Model file for the job. Use its own axes, mm. A direction names the side the tool comes from. Round coordinates to 2 decimals unless told otherwise and drop trailing zeros. Loops run counter-clockwise (first coordinate to the right, second up) from the corner with the lowest first, then second, coordinate; pieces in that order, holes last. Notation, with made-up numbers: (-2.75, 22) - (12.25, 22) arc R14 cw to (12.25, 42) - close; hole circle Ø8 at (-11.5, 54.25). An arc over 180 degrees is marked (long way). Answer as a JSON object with one key per item and string values.
from build123d import *

# Parameters (mm, degrees)
SKETCH1_W                   = 76.1
SKETCH1_H                   = 151.5
BOSS_EXTRUDE2_DEPTH         = 8
SKETCH1_4_W                 = 76.1
SKETCH1_4_H                 = 3
BOSS_EXTRUDE3_DEPTH         = 18.5
CUT_EXTRUDE_THIN1_START     = -8
CUT_EXTRUDE_THIN1_OUTLINE_W = 50
CUT_EXTRUDE_THIN1_OUTLINE_H = 4.46993239
CUT_EXTRUDE_THIN1_DEPTH     = 18.5
SKETCH4_W                   = 76.1
SKETCH4_H                   = 3
CUT_EXTRUDE1_DEPTH          = 16.5
SKETCH6_W                   = 154.5
SKETCH6_H                   = 2
BOSS_EXTRUDE4_DEPTH         = 3
SKETCH7_W                   = 154.5
SKETCH7_H                   = 2
BOSS_EXTRUDE5_DEPTH         = 3
CUT_EXTRUDE2_DEPTH          = 3
CUT_EXTRUDE2_DEPTH_BACK     = 76.1
SKETCH8_R                   = 1.75


# Read off the part's stored shape, not the designer's step: Cut-Extrude-Thin1
with BuildPart() as part:
    # Sketch1 → Boss-Extrude2 (new body)
    with BuildSketch(Plane(origin=(0, 0, 0), x_dir=(1, 0, 0), z_dir=(0, 1, 0))):
        with Locations((38.05, -75.75)):
            Rectangle(SKETCH1_W, SKETCH1_H)
    extrude(amount=BOSS_EXTRUDE2_DEPTH)

    # Sketch1<4> → Boss-Extrude3 (add)
    with BuildSketch(Plane(origin=(0, 0, 0), x_dir=(1, 0, 0), z_dir=(0, 1, 0))):
        Polygon((0, -151.5), (-3, -151.5), (-3, -155.96993239), (79.1, -155.96993239), (79.1, -151.5), (76.1, -151.5), align=None)
        Polygon((0, 3), (-3, 3), (-3, -151.5), (0, -151.5), (0, 0), align=None)
        Polygon((79.1, 3), (79.1, -151.5), (76.1, -151.5), (76.1, 0), (76.1, 3), align=None)
        with Locations((38.05, 1.5)):
            Rectangle(SKETCH1_4_W, SKETCH1_4_H)
    extrude(amount=BOSS_EXTRUDE3_DEPTH)

    # Cut-Extrude-Thin1 outline → Cut-Extrude-Thin1 (cut)
    with BuildSketch(Plane(origin=(0, 8, 0), x_dir=(1, 0, 0), z_dir=(0, 1, 0)).offset(CUT_EXTRUDE_THIN1_START)):
        with Locations((38.05, -153.734966195)):
            Rectangle(CUT_EXTRUDE_THIN1_OUTLINE_W, CUT_EXTRUDE_THIN1_OUTLINE_H)
    extrude(amount=CUT_EXTRUDE_THIN1_DEPTH, mode=Mode.SUBTRACT)

    # Sketch4 → Cut-Extrude1 (cut)
    with BuildSketch(Plane(origin=(0, 18.5, 0), x_dir=(1, 0, 0), z_dir=(0, 1, 0))):
        with Locations((38.05, 1.5)):
            Rectangle(SKETCH4_W, SKETCH4_H)
    extrude(amount=-CUT_EXTRUDE1_DEPTH, mode=Mode.SUBTRACT)

    # Sketch6 → Boss-Extrude4 (add)
    with BuildSketch(Plane(origin=(0, 0, 0), x_dir=(0, 0, -1), z_dir=(1, 0, 0))):
        with Locations((-74.25, 17.5)):
            Rectangle(SKETCH6_W, SKETCH6_H)
    extrude(amount=BOSS_EXTRUDE4_DEPTH)

    # Sketch7 → Boss-Extrude5 (add)
    with BuildSketch(Plane.ZY.offset(-76.1)):
        with Locations((74.25, 17.5)):
            Rectangle(SKETCH7_W, SKETCH7_H)
    extrude(amount=BOSS_EXTRUDE5_DEPTH)

    # Sketch8 → Cut-Extrude2 (cut, two sides: drawn at the far end of the back side and taken through both)
    with BuildSketch(Plane(origin=(0, 8, 0), x_dir=(1, 0, 0), z_dir=(0, 1, 0)).offset(-CUT_EXTRUDE2_DEPTH_BACK)):
        with Locations(Location((38.05, -75.75, 0), (0, 0, 270))):
            Circle(SKETCH8_R)
    extrude(amount=CUT_EXTRUDE2_DEPTH + CUT_EXTRUDE2_DEPTH_BACK, mode=Mode.SUBTRACT)


solid = part.part
1) Slice it at D-D on x = 24. List the corners of the cut face in (y, z), then the cut area to 3 significant figures.
Values follow:
{"outline": "(0, -3) - (2, -3) - (2, 0) - (8, 0) - (8, 151.5) - (0, 151.5) - close", "area": "1,220 mm²"}
2) Tool access for faces 1 (the flat face through (38.2, 1.7, -3)), 2 (the flat face through (0, 13, 75)), 3 (the flat face through (13.05, 9, 154)): list every direction of +Z, -Z, +X, -X, +Y, -Y with a clear straight run to the whole face (end or side of a thin tool).
Values follow:
{"face 1": "-Z, +X, -X, +Y, -Y", "face 2": "-Z", "face 3": "+Z, +Y, -Y"}
3) Drop flat-ended pins along their axis: P1, Ø3.5, axis at x = 56.5, z = -1.5, coming from the +Y side; P2, Ø6.5, axis at x = 37, y = 4, coming from the +Z side; P3, Ø1.8, axis at x = 24, y = 4, coming from the -Z side. Give the stop position or say it passes through.
Values follow:
{"P1": "y = 8", "P2": "z = 151.5", "P3": "z = 0"}
4) Slice it at A-A on z = 75.75. List the corners of the cut face in (x, y), then the cut area to 3 significant figures.
Values follow:
{"outline": "(-3, 0) - (36.3, 0) - (36.3, 8) - (0, 8) - (0, 16.5) - (3, 16.5) - (3, 18.5) - (-3, 18.5) - close; (39.8, 0) - (79.1, 0) - (79.1, 18.5) - (73.1, 18.5) - (73.1, 16.5) - (76.1, 16.5) - (76.1, 8) - (39.8, 8) - close", "area": "704 mm²"}
5) Slice it at C-C on x = 38.05. List the corners of the cut face in (y, z).
Values follow:
{"outline": "(0, -3) - (2, -3) - (2, 0) - (8, 0) - (8, 74) - (0, 74) - close; (0, 77.5) - (8, 77.5) - (8, 151.5) - (0, 151.5) - close"}
6) Probe probe 1 along X at (y, z) = (10.5, 111); probe 2 along X at (y, z) = (4.75, 75.75); probe 3 along Y at (x, z) = (74.5, 139). List the from-to ranges inside material, lowest first.
Values follow:
{"probe 1": "-3 to 0, 76.1 to 79.1", "probe 2": "-3 to 36.3, 39.8 to 79.1", "probe 3": "0 to 8, 16.5 to 18.5"}
7) Slice it at B-B on y = 10.5. List the corners of the cut face in (x, z).
Values follow:
{"outline": "(-3, -3) - (0, -3) - (0, 151.5) - (13.05, 151.5) - (13.05, 155.97) - (-3, 155.97) - close; (63.05, 151.5) - (76.1, 151.5) - (76.1, -3) - (79.1, -3) - (79.1, 155.97) - (63.05, 155.97) - close"}
8) Two-plate mould, pull along Y, no slides. Class faces 4 (the cylindrical face through (38.576, 3.944, 77.419)), 5 (the flat face through (75, 16.5, 73)), 6 (the flat face through (76, 18.5, 82)): pulls with the +Y half, pulls with the -Y half, needs draft (parallel to the pull), parting line crosses it, or undercut.
Values follow:
{"face 4": "needs draft", "face 5": "undercut", "face 6": "pulls with the +Y half"}
